Part model, mm, in its own coordinate system. A direction names the side the tool comes from. Give positions to 0.01 mm unless a question says otherwise; leave off trailing zeros. Write each loop counter-clockwise with the first axis right and the second up, starting at its lowest first coordinate (ties: lowest second). Pieces come first, ordered by that corner, then holes. Notation, with made-up numbers: M -32,5.25 L 16,5.25 A17 ccw 16,10.25 Z; hole C 86,42.25 d8. An arc over 180 degrees is marked long. Use CSV: the item, a comma, the result in double quotes. Start each with the question number.
1. Band-saw the part on A-A, the plane y = 1.5. List the corners of the cut face in (x, z), then the cut area to 3 significant figures.
2. Drill centre lines: line 1 along Z through (x, y) = (214.5, -2.5); line 2 along X through (y, z) = (4.75, -2.25). Where is each one in solid material? Low to high. Write a range as from..to.
3. Drop a flat-ended pin along its axis: pin 1 Ø1.5 at (x, z) = (-173, 2) entering from -Y. Give the stop position or say it passes through.
4. 3-axis set-ups, long thin cutter, end or side, ignore diameter. For faces 1 (the face through (-299, -1, 0)), 2 (the face through (-300, 0, 0)): which of +Z, -Z, +X, -X, +Y, -Y reach the whole face in a straight line?
5. Band-saw the part on B-B, the plane x = -145. List the corners of the cut face in (y, z), then the cut area to 3 significant figures.
6. Band-saw the part on C-C, the plane z = 0. List the corners of the cut face in (x, y), then the cut area to 3 significant figures.
7. Mould opens along Y. For faces 3 (the face through (4, 0, -7.5)), 4 (the face through (4, 5.5, 0)), 5 (the face through (4, 7.5, 0)), 6 (the face through (4, -7.5, -5)) say: pulls with the +Y half, pulls with the -Y half, needs draft (parallel to the pull), parting line crosses it, or undercut.
from build123d import *

# Parameters (mm, degrees)
F1_DEPTH = 299
F3_W     = 15
F3_H     = 15
F4_DEPTH = 1
F6_W     = 15
F6_H     = 15
F7_DEPTH = 1


# Not quite as in the source:
# - the program builds the solid bodies; features that only make, move or delete a surface that nothing else refers to are left out


with BuildPart() as f1:
    # F0 (on Right) → F1 (new body, symmetric)
    with BuildSketch(Plane.YZ):
        Polygon((7.5, 7.5), (-7.5, 7.5), (-7.5, 3.5), (-5.5, 3.5), (-5.5, 5.5), (5.5, 5.5), (5.5, -5.5), (-5.5, -5.5), (-5.5, -3.5), (-7.5, -3.5), (-7.5, -7.5), (7.5, -7.5), align=None)
    extrude(amount=F1_DEPTH, both=True)

    # F3 (on offset) → F4 (join)
    with BuildSketch(Plane.YZ.offset(299)):
        Rectangle(F3_W, F3_H)
    extrude(amount=F4_DEPTH)

    # F6 (on offset) → F7 (join)
    with BuildSketch(Plane(origin=(-299, 0, 0), x_dir=(0, -1, 0), z_dir=(-1, 0, 0))):
        Rectangle(F6_W, F6_H)
    extrude(amount=F7_DEPTH)


solid = f1.part
Output:
1,outline,"M -300,-7.5 L 300,-7.5 L 300,7.5 L -300,7.5 Z; hole M -299,-5.5 L 299,-5.5 L 299,5.5 L -299,5.5 Z"
1,area,"2,420 mm²"
2,line 1,"z = -7.5..-5.5, 5.5..7.5"
2,line 2,"x = -300..-299, 299..300"
3,pin 1,"stops at y = 5.5"
4,face 1,"none"
4,face 2,"+Z, -Z, -X, +Y, -Y"
5,outline,"M -7.5,-7.5 L 7.5,-7.5 L 7.5,7.5 L -7.5,7.5 L -7.5,3.5 L -5.5,3.5 L -5.5,5.5 L 5.5,5.5 L 5.5,-5.5 L -5.5,-5.5 L -5.5,-3.5 L -7.5,-3.5 Z"
5,area,"90.0 mm²"
6,outline,"M -300,-7.5 L -299,-7.5 L -299,5.5 L 299,5.5 L 299,-7.5 L 300,-7.5 L 300,7.5 L -300,7.5 Z"
6,area,"1,230 mm²"
7,face 3,"needs draft"
7,face 4,"undercut"
7,face 5,"pulls with the +Y half"
7,face 6,"pulls with the -Y half"
